```python
from build123d import *

# Parameters (mm, degrees)
SKETCH1_W           = 127
SKETCH1_H           = 87
BOSS_EXTRUDE1_DEPTH = 1.5
SKETCH2_W           = 131
SKETCH2_H           = 91
SKETCH2_W_2         = 127
SKETCH2_H_2         = 87
BOSS_EXTRUDE2_DEPTH = 10
CUT_EXTRUDE1_REACH  = 82.377
SKETCH3_W           = 44
SKETCH3_H           = 4
SKETCH5_W           = 129
SKETCH5_H           = 89
SKETCH5_W_2         = 127
SKETCH5_H_2         = 87
CUT_EXTRUDE3_DEPTH  = 1.5


with BuildPart() as part:
    # Sketch1 → Boss-Extrude1 (new body)
    with BuildSketch(Plane(origin=(0, 0, 0), x_dir=(1, 0, 0), z_dir=(0, 1, 0))):
        Rectangle(SKETCH1_W, SKETCH1_H)
    extrude(amount=BOSS_EXTRUDE1_DEPTH)

    # Sketch2 → Boss-Extrude2 (add)
    with BuildSketch(Plane(origin=(0, 0, 0), x_dir=(1, 0, 0), z_dir=(0, 1, 0))):
        Rectangle(SKETCH2_W, SKETCH2_H)
        Rectangle(SKETCH2_W_2, SKETCH2_H_2, mode=Mode.SUBTRACT)
    extrude(amount=BOSS_EXTRUDE2_DEPTH)

    # Sketch3 → Cut-Extrude1 (cut, up to next)
    with BuildSketch(Plane.XZ, mode=Mode.PRIVATE) as cut_extrude1_sk1:
        with Locations((-16.5, 30.5)):
            Rectangle(SKETCH3_W, SKETCH3_H)
    cut_extrude1_tool1 = extrude(cut_extrude1_sk1.sketch, amount=-CUT_EXTRUDE1_REACH, mode=Mode.PRIVATE) & part.part
    add(cut_extrude1_tool1.solids().sort_by_distance((-16.5, 0, 30.5))[0], mode=Mode.SUBTRACT)

    # Sketch5 → Cut-Extrude3 (cut)
    with BuildSketch(Plane(origin=(0, 10, 0), x_dir=(1, 0, 0), z_dir=(0, 1, 0))):
        Rectangle(SKETCH5_W, SKETCH5_H)
        Rectangle(SKETCH5_W_2, SKETCH5_H_2, mode=Mode.SUBTRACT)
    extrude(amount=-CUT_EXTRUDE3_DEPTH, mode=Mode.SUBTRACT)


solid = part.part
```
Source: CAD feature listing. Evaluate the final solid. Frame: model axes, mm. A direction names the side the tool comes from. Coordinates: 2 decimals unless noted, no trailing zeros. Write each loop counter-clockwise with the first axis right and the second up, starting at its lowest first coordinate (ties: lowest second). Pieces come first, ordered by that corner, then holes. Notation, with made-up numbers: (31.5, 23.25) -> (47.5, 23.25) arc R32 ccw to (47.5, 56.25) -> close; hole circle Ø4 at (89.5, 50). An arc over 180 degrees is marked (long way). Return JSON: item names as keys, results as strings. Group by question number.
1) Section query A-A, the plane x = -17.5. Return loops of the section in (y, z), plus the area to 4 significant figures.
2) Set-up query: faces 5 (the face through (-1, 1.5, -1)), 6 (the face through (65.5, 5, 1)). Return all of +Z, -Z, +X, -X, +Y, -Y with unobstructed straight access to the full face (end or side cutting, diameter ignored); none if empty.
3) Section query C-C, the plane z = 30. Return loops of the section in (x, y).
4) Section query B-B, the plane y = 5. Return loops of the section in (x, z), plus the area to 3 significant figures.
5) Section query D-D, the plane x = 19. Return loops of the section in (y, z), plus the area to 4 significant figures.
6) Mould query, pull axis Z, two halves, no side actions, for faces 1 (the face through (-1, 5, 45.5)), 2 (the face through (-1, 5, -45.5)), 3 (the face through (-1, 5, -43.5)), 4 (the face through (-63.5, 5, 1)). Classes: +Z half, -Z half, draft (parallel to the pull), parting line (faces both ways), or undercut.
7) Ray query, line 1 along Z through (x, y) = (54.5, 4); line 2 along X through (y, z) = (8.25, 6); line 3 along Z through (x, y) = (-7, 9.5). Return the intervals inside material, ascending.
8) Contact query for a flat-ended pin moving along its axis: P1, Ø10, axis at x = -46.5, z = -4.5, coming from the +Y side. Output: stop coordinate, or through.
From the geometry:
{
 "1": {"outline": "(0, -45.5) -> (10, -45.5) -> (10, -44.5) -> (8.5, -44.5) -> (8.5, -43.5) -> (1.5, -43.5) -> (1.5, 28.5) -> (0, 28.5) -> close; (0, 32.5) -> (1.5, 32.5) -> (1.5, 43.5) -> (8.5, 43.5) -> (8.5, 44.5) -> (10, 44.5) -> (10, 45.5) -> (0, 45.5) -> close", "area": "161.5 mm²"},
 "2": {"face 5": "+Y", "face 6": "+Z, -Z, +X, +Y, -Y"},
 "3": {"outline": "(-65.5, 0) -> (-38.5, 0) -> (-38.5, 1.5) -> (-63.5, 1.5) -> (-63.5, 8.5) -> (-64.5, 8.5) -> (-64.5, 10) -> (-65.5, 10) -> close; (5.5, 0) -> (65.5, 0) -> (65.5, 10) -> (64.5, 10) -> (64.5, 8.5) -> (63.5, 8.5) -> (63.5, 1.5) -> (5.5, 1.5) -> close"},
 "4": {"outline": "(-65.5, -45.5) -> (65.5, -45.5) -> (65.5, 45.5) -> (-65.5, 45.5) -> close; hole (-63.5, -43.5) -> (63.5, -43.5) -> (63.5, 43.5) -> (-63.5, 43.5) -> close", "area": "872 mm²"},
 "5": {"outline": "(0, -45.5) -> (10, -45.5) -> (10, -44.5) -> (8.5, -44.5) -> (8.5, -43.5) -> (1.5, -43.5) -> (1.5, 43.5) -> (8.5, 43.5) -> (8.5, 44.5) -> (10, 44.5) -> (10, 45.5) -> (0, 45.5) -> close", "area": "167.5 mm²"},
 "6": {"face 1": "+Z half", "face 2": "-Z half", "face 3": "undercut", "face 4": "undercut"},
 "7": {"line 1": "-45.5 to -43.5, 43.5 to 45.5", "line 2": "-65.5 to -63.5, 63.5 to 65.5", "line 3": "-45.5 to -44.5, 44.5 to 45.5"},
 "8": {"P1": "y = 1.5"}
}
